Here's how the part is built. I have some questions about the finished solid (model axes, mm). Give positions to 0.01 mm unless a question says otherwise; leave off trailing zeros. Order: outer loops, then holes, each group sorted by start corner. A loop starts at its lowest first (then second) coordinate and runs counter-clockwise, first axis right, second up. Notation, with made-up numbers: M 68.25,-13 L 121.25,-13 A23 cw 121.25,16 Z; hole C 54.25,-10.75 d1. An arc over 180 degrees is marked long. Use one line per item in the form item = value.
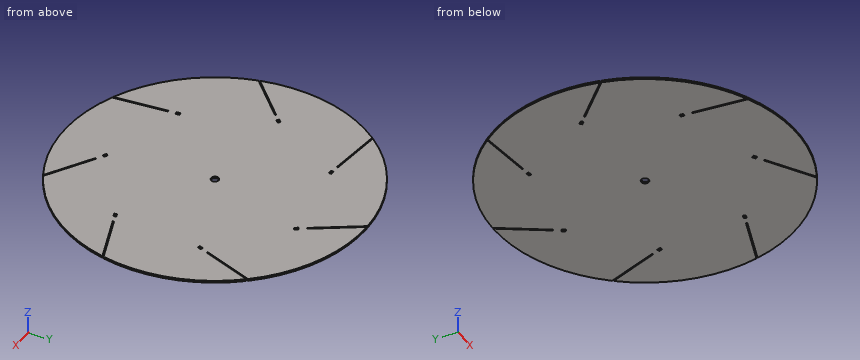
from build123d import *

# Parameters (mm, degrees)
F0_R          = 5
F1_DEPTH      = 1.25
F1_DEPTH_BACK = 1.25


with BuildPart() as f1:
    # F0 (on Top) → F1 (new body, two sides)
    with BuildSketch(Plane.XY) as f1_sk:
        with BuildLine():
            Line((-193.64496, -48.269231), (-144.827721, 0.548008))
            Line((-144.827721, 0.548008), (-143.731706, -0.548008))
            Line((-143.731706, -0.548008), (-193.552665, -50.368296))
            ThreePointArc((-193.552665, -50.368296), (-153.272634, -128.48028), (-83.395599, -181.782841))
            Line((-83.395599, -181.782841), (-82.996864, -181.493909))
            Line((-82.996864, -181.493909), (-90.726667, -112.890004))
            Line((-90.726667, -112.890004), (-89.186413, -112.716459))
            Line((-89.186413, -112.716459), (-81.298203, -182.730495))
            ThreePointArc((-81.298203, -182.730495), (4.886394, -199.940324), (90.127633, -178.541862))
            Line((90.127633, -178.541862), (90.150343, -178.049972))
            Line((90.150343, -178.049972), (31.694198, -141.319541))
            Line((31.694198, -141.319541), (32.518847, -140.007118))
            Line((32.518847, -140.007118), (92.176243, -177.492904))
            ThreePointArc((92.176243, -177.492904), (159.366647, -120.841226), (195.783698, -40.855219))
            Line((195.783698, -40.855219), (195.413283, -40.530774))
            Line((195.413283, -40.530774), (130.249465, -63.33258))
            Line((130.249465, -63.33258), (129.737532, -61.869561))
            Line((129.737532, -61.869561), (196.240878, -38.599537))
            ThreePointArc((196.240878, -38.599537), (193.841344, 49.25378), (154.011425, 127.596237))
            Line((154.011425, 127.596237), (153.526814, 127.508923))
            Line((153.526814, 127.508923), (130.725008, 62.345105))
            Line((130.725008, 62.345105), (129.261989, 62.857037))
            Line((129.261989, 62.857037), (152.532909, 129.360069))
            ThreePointArc((152.532909, 129.360069), (82.350335, 182.259685), (-3.733812, 199.965124))
            Line((-3.733812, 199.965124), (-3.967697, 199.5318))
            Line((-3.967697, 199.5318), (32.762734, 141.075654))
            Line((32.762734, 141.075654), (31.450311, 140.251005))
            Line((31.450311, 140.251005), (-6.034672, 199.908905))
            ThreePointArc((-6.034672, 199.908905), (-91.151376, 178.02033), (-158.666634, 121.756194))
            Line((-158.666634, 121.756194), (-158.473672, 121.303162))
            Line((-158.473672, 121.303162), (-89.869768, 113.573359))
            Line((-89.869768, 113.573359), (-90.043313, 112.033105))
            Line((-90.043313, 112.033105), (-160.057242, 119.922257))
            ThreePointArc((-160.057242, 119.922257), (-196.013462, 39.728035), (-194.119464, -48.137634))
            Line((-194.119464, -48.137634), (-193.64496, -48.269231))
        make_face()
        Polygon((-91.636007, -97.897549), (-89.872168, -97.698812), (-89.312346, -102.667373), (-91.076185, -102.86611), (-92.840024, -103.064847), (-93.399847, -98.096286), align=None, mode=Mode.SUBTRACT)
        Circle(F0_R, mode=Mode.SUBTRACT)
        Polygon((19.405659, -132.682848), (20.350016, -131.179913), (24.583637, -133.840073), (23.63928, -135.343009), (22.694924, -136.845944), (18.461303, -134.185784), align=None, mode=Mode.SUBTRACT)
        Polygon((115.835249, -67.555257), (115.249003, -65.879864), (119.96842, -64.228469), (120.554665, -65.903862), (121.140911, -67.579254), (116.421494, -69.23065), align=None, mode=Mode.SUBTRACT)
        Polygon((-137.208646, 7.071068), (-138.46376, 8.326182), (-134.928226, 11.861716), (-133.673112, 10.606602), (-132.417997, 9.351487), (-135.953531, 5.815953), align=None, mode=Mode.SUBTRACT)
        Polygon((-75.050857, 111.123765), (-75.249594, 109.359926), (-80.218155, 109.919748), (-80.019418, 111.683587), (-79.820681, 113.447426), (-74.85212, 112.887604), align=None, mode=Mode.SUBTRACT)
        Polygon((125.039313, 48.442821), (123.36392, 49.029066), (125.015315, 53.748483), (126.690708, 53.162238), (128.366101, 52.575992), (126.714706, 47.856576), align=None, mode=Mode.SUBTRACT)
        Polygon((40.087004, 127.962466), (38.584068, 127.01811), (35.923908, 131.251731), (37.426843, 132.196087), (38.929779, 133.140444), (41.589939, 128.906823), align=None, mode=Mode.SUBTRACT)
    extrude(amount=F1_DEPTH)
    extrude(f1_sk.sketch, amount=-F1_DEPTH_BACK)


solid = f1.part
Q1. I want a section at C-C on x = 78. Write out the boundary of the cut face in (y, z).
Found:
outline = M -184.16,-1.25 L -170.42,-1.25 L -170.42,1.25 L -184.16,1.25 Z; M -168.59,-1.25 L 184.16,-1.25 L 184.16,1.25 L -168.59,1.25 Z
Q2. I want a section at A-A on x = 168.5. Write out the boundary of the cut face in (y, z), then the cut area to 3 significant figures.
Found:
outline = M -107.74,-1.25 L -49.95,-1.25 L -49.95,1.25 L -107.74,1.25 Z; M -48.31,-1.25 L 107.74,-1.25 L 107.74,1.25 L -48.31,1.25 Z
area = 535 mm²
Q3. I want a section at D-D on x = -64. Write out the boundary of the cut face in (y, z).
Found:
outline = M -189.48,-1.25 L 189.48,-1.25 L 189.48,1.25 L -189.48,1.25 Z
Q4. I'm going to push a flat-ended pin straight in: pin 1 Ø1.5 at (y, z) = (10.5, 0) entering from -X. Where does the tip first touch, or does it pass through?
Found:
pin_1 = -199.76
Q5. I need wall thicknesses on L1, parallel to Y at x = 0, z = 0; L2, parallel to X at y = -3, z = 0.8; L3, parallel to X at y = -179.5, z = 0.25. Which ranges of each line are inside material? Lowest first, please.
Found:
L1 = -200 to -5, 5 to 190.3, 193.22 to 200
L2 = -199.98 to -148.38, -146.18 to -4, 4 to 199.98
L3 = -88.2 to -83.22, -81.66 to 88.2
Q6. I want a section at B-B on z = -0.2. State how many separate pieces and enclosed holes the cut face has, then the cut area to 3 significant figures.
Found:
separate_pieces = 1
enclosed_holes = 8
area = 125,000 mm²
